from build123d import *

# Parameters (mm, degrees)
SKETCH3_R               = 21.59
GEARBODY_DEPTH          = 25.4
TOOTHCUT_DEPTH          = 40.716699259
CIRPATTERN1_COUNT       = 15
BOREDIA_R               = 9.525
BORE_DEPTH              = 12700
CUT_EXTRUDE1_DEPTH      = 40.703986775
CUT_EXTRUDE1_DEPTH_BACK = 40.703986775


with BuildPart() as part:
    # Sketch3 → gearBody (new body)
    with BuildSketch(Plane.XY):
        Circle(SKETCH3_R)
    extrude(amount=GEARBODY_DEPTH)

    # Sketch2 → toothCut (cut, through all)
    with BuildSketch(Plane.XY):
        with BuildLine():
            ThreePointArc((15.783846764, -2.304552616), (15.843293638, -1.852249483), (15.889781974, -1.39843136))
            ThreePointArc((15.889781974, -1.39843136), (16.213055843, -0.751556907), (16.890861518, -0.499501321))
            ThreePointArc((16.890861518, -0.499501321), (20.504912911, 0.340315353), (23.283949955, 2.798691365))
            ThreePointArc((23.283949955, 2.798691365), (23.292901215, -2.723187818), (22.010467945, -8.09409042))
            ThreePointArc((22.010467945, -8.09409042), (19.873444675, -5.060974685), (16.550574786, -3.410158156))
            ThreePointArc((16.550574786, -3.410158156), (15.949189176, -3.008551507), (15.783846764, -2.304552616))
        make_face()
    toothcut = extrude(amount=TOOTHCUT_DEPTH, mode=Mode.SUBTRACT)

    # CirPattern1: toothCut ×15 about axis
    cirpattern1_axis = Axis((0, 0, 0), (0, 0, 1))
    for i in range(1, CIRPATTERN1_COUNT):
        add(toothcut.rotate(cirpattern1_axis, i * 360 / CIRPATTERN1_COUNT), mode=Mode.SUBTRACT)

    # boreDia → bore (cut, symmetric)
    with BuildSketch(Plane.XY):
        Circle(BOREDIA_R)
    extrude(amount=BORE_DEPTH, both=True, mode=Mode.SUBTRACT)

    # Sketch4 → Cut-Extrude1 (cut, two sides: drawn at the far end of the back side and taken through both)
    with BuildSketch(Plane(origin=(0, 0, 0), x_dir=(0, 0, -1), z_dir=(1, 0, 0)).offset(-CUT_EXTRUDE1_DEPTH_BACK)):
        Polygon((-3.81, 26.191979423), (-3.81, -31.870423863), (6.096210589, -32.468383172), (8.920928288, 23.481458771), align=None)
    extrude(amount=CUT_EXTRUDE1_DEPTH + CUT_EXTRUDE1_DEPTH_BACK, mode=Mode.SUBTRACT)


solid = part.part
Geometry check sheet. Reference: the model listing, model coordinates, mm. A direction names the side the tool comes from. Give positions to 0.01 mm unless a question says otherwise; leave off trailing zeros. Answer as a JSON object with one key per item and string values. Group by question number.
Item 1: Gauge pin test, flat ends, axial feed: pin 1 (1 mm diameter, centred on y = -9.5, z = 15.5, fed in from -X); pin 2 (6 mm diameter, centred on x = 16, z = 19.5, fed in from +Y). Record the tip position at first contact, or that the pin passes through.
Item 2: Material ranges on L1, parallel to Y at x = 18.5, z = 21.5; L2, parallel to Y at x = 0, z = 8.75 (3 decimals); L3, parallel to Y at x = 18, z = 17.25, recorded low to high.
Item 3: Access from +Z, -Z, +X, -X, +Y, -Y to the whole of each face (thin tool, end or side, straight path). Record for faces 1 (the cylindrical face through (15.492, -11.658, 14.454)), 2 (the cylindrical face through (-15.544, 11.477, 14.454)), 3 (the cylindrical face through (-11.135, 11.819, 14.454)).
Item 4: Mould release check, pull along Y, two halves, no side actions. Record for faces 4 (the cylindrical face through (8.434, -13.876, 14.454)), 5 (the cylindrical face through (18.83, 10.56, 14.45)), 6 (the cylindrical face through (8.54, -19.83, 14.45)), 7 (the cylindrical face through (-14.98, 6.27, 14.45)): pulls with the +Y half, pulls with the -Y half, needs draft (parallel to the pull), parting line crosses it, or undercut.
Findings below:
{
 "1": {"pin 1": "x = -14.57", "pin 2": "y = 17.24"},
 "2": {"L1": "-8.04 to -4.12, -0.36 to 3.76, 8.54 to 11.13", "L2": "-21.59 to -9.525, 9.525 to 15.951", "L3": "-8.03 to -3.88, -0.44 to 3.78, 7.99 to 11.44"},
 "3": {"face 1": "+Z, -Z, +X", "face 2": "+Z, -Z, +Y", "face 3": "+Z, -Z"},
 "4": {"face 4": "undercut", "face 5": "pulls with the +Y half", "face 6": "pulls with the -Y half", "face 7": "undercut"}
}
